Part model, mm, in its own coordinate system. A direction names the side the tool comes from. Give positions to 0.01 mm unless a question says otherwise; leave off trailing zeros. Order: outer loops, then holes, each group sorted by start corner. A loop starts at its lowest first (then second) coordinate and runs counter-clockwise, first axis right, second up.
from build123d import *

# Parameters (mm, degrees)
BOSS_EXTRUDE1_DEPTH   = 5.588
F_6_CLEARANCE_HOLE1_D = 3.7973
M2_CLEARANCE_HOLE1_D  = 2.4
CUT_EXTRUDE1_REACH    = 254.133
SKETCH8_R             = 5.08


with BuildPart() as part:
    # Sketch1 → Boss-Extrude1 (new body)
    with BuildSketch(Plane(origin=(0, 0, 0), x_dir=(1, 0, 0), z_dir=(0, 1, 0))):
        with BuildLine():
            Line((12.7, 72.898), (31.75, 72.898))
            Line((31.75, 72.898), (31.75, 67.056))
            Line((31.75, 67.056), (44.45, 67.056))
            Line((44.45, 67.056), (44.45, 72.898))
            Line((44.45, 72.898), (69.85, 72.898))
            Line((69.85, 72.898), (69.85, 67.31))
            Line((69.85, 67.31), (114.3, 67.31))
            Line((114.3, 67.31), (114.3, 72.898))
            Line((114.3, 72.898), (139.7, 72.898))
            Line((139.7, 72.898), (139.7, 67.31))
            Line((139.7, 67.31), (165.1, 67.31))
            Line((165.1, 67.31), (165.1, 72.898))
            Line((165.1, 72.898), (190.5, 72.898))
            Line((190.5, 72.898), (190.5, 67.056))
            Line((190.5, 67.056), (222.25, 67.056))
            Line((222.25, 67.056), (222.25, 72.898))
            Line((222.25, 72.898), (241.3, 72.898))
            Line((241.3, 72.898), (241.3, 0))
            Line((241.3, 0), (171.45, 0))
            ThreePointArc((171.45, 0), (162.469743879, -3.719743879), (158.75, -12.7))
            Line((158.75, -12.7), (158.75, -42.164))
            Line((158.75, -42.164), (146.05, -42.164))
            Line((146.05, -42.164), (146.05, 0.122766638))
            Line((146.05, 0.122766638), (127, 0.122766638))
            Line((127, 0.122766638), (107.95, 0.122766638))
            Line((107.95, 0.122766638), (107.95, -42.164))
            Line((107.95, -42.164), (95.25, -42.164))
            Line((95.25, -42.164), (95.25, -12.7))
            ThreePointArc((95.25, -12.7), (91.530256121, -3.719743879), (82.55, 0))
            Line((82.55, 0), (12.7, 0))
            Line((12.7, 0), (12.7, 72.898))
        make_face()
    extrude(amount=BOSS_EXTRUDE1_DEPTH)

    # #6 Clearance Hole1 (through all)
    with Locations(Plane(origin=(0, 0, 0), x_dir=(-1, 0, 0), z_dir=(0, -1, 0))):
        with Locations((-102.362, -32.397617544), (-151.638, -32.397617544), (-151.638, -5.456849181), (-102.362, -5.456849181)):
            Hole(F_6_CLEARANCE_HOLE1_D / 2)

    # M2 Clearance Hole1 (through all)
    with Locations(Plane(origin=(0, 5.588, 0), x_dir=(1, 0, 0), z_dir=(0, 1, 0))):
        with Locations((33.528, 58.166), (53.848, 58.166), (53.848, 37.846), (33.528, 37.846)):
            Hole(M2_CLEARANCE_HOLE1_D / 2)

    # Sketch8 → Cut-Extrude1 (cut, up to next)
    with BuildSketch(Plane(origin=(0, 5.588, 0), x_dir=(1, 0, 0), z_dir=(0, 1, 0)), mode=Mode.PRIVATE) as cut_extrude1_sk1:
        with Locations(Location((28.448, 15.870766638, 0), (0, 0, 270))):
            Circle(SKETCH8_R)
    cut_extrude1_tool1 = extrude(cut_extrude1_sk1.sketch, amount=-CUT_EXTRUDE1_REACH, mode=Mode.PRIVATE) & part.part
    # Sketch8 → Cut-Extrude1 (cut, up to next)
    with BuildSketch(Plane(origin=(0, 5.588, 0), x_dir=(1, 0, 0), z_dir=(0, 1, 0)), mode=Mode.PRIVATE) as cut_extrude1_sk2:
        with Locations(Location((225.552, 15.870766638, 0), (0, 0, 270))):
            Circle(SKETCH8_R)
    cut_extrude1_tool2 = extrude(cut_extrude1_sk2.sketch, amount=-CUT_EXTRUDE1_REACH, mode=Mode.PRIVATE) & part.part
    add(cut_extrude1_tool1.solids().sort_by_distance((28.448, 5.588, -15.870767))[0], mode=Mode.SUBTRACT)
    add(cut_extrude1_tool2.solids().sort_by_distance((225.552, 5.588, -15.870767))[0], mode=Mode.SUBTRACT)


solid = part.part
Item 1: Pull direction Z, two halves, no side cores. Call faces 1 (the face through (31.9, 2.8, -19.6)), 2 (the face through (241.3, 3, -37)), 3 (the face through (48, 3, 0)): released by +Z, released by -Z, zero draft, split by the parting line, or undercut.
Item 2: Drill centre lines: probe 1 along X at (y, z) = (2.9, -57.5); probe 2 along X at (y, z) = (1.95, 35.5); probe 3 along X at (y, z) = (5, -17.5). Where is each one in solid material? Low to high.
Item 3: Band-saw the part on B-B on x = 144. List the corners of the cut face in (y, z), plus the area to 3 significant figures.
Item 4: Band-saw the part on C-C on y = 3. Give the number of separate pieces and of enclosed holes in the cut face, plus the area to 3 significant figures.
Item 5: Which spindle directions (+Z, -Z, +X, -X, +Y, -Y) get a long thin tool onto all of the face, cutting with end or side? Do faces 4 (the face through (207, 3, 0)), 5 (the face through (31.75, 3, -70)), 6 (the face through (146.05, 3, 21)). Say none if no direction does.
Item 6: Band-saw the part on D-D on x = 118. List the corners of the cut face in (y, z), plus the area to 3 significant figures.
Item 7: Drop flat-ended pins along their axis: P1, Ø3, axis at x = 203, y = 4, coming from the +Z side; P2, Ø1.7, axis at x = 36.5, y = 1.5, coming from the -Z side; P3, Ø3, axis at y = 2, z = 31.5, coming from the -X side. Give the stop position or say it passes through.
Item 8: Band-saw the part on A-A on z = 18.5. List the corners of the cut face in (x, y), plus the area to 3 significant figures.
Working result:
1. face 1: undercut
1. face 2: zero draft
1. face 3: released by +Z
2. probe 1: x = 12.7 to 32.53, 34.53 to 52.85, 54.85 to 241.3
2. probe 2: x = 95.25 to 107.95, 146.05 to 158.75
2. probe 3: x = 12.7 to 23.64, 33.26 to 220.74, 230.36 to 241.3
3. outline: (0, -67.31) - (5.59, -67.31) - (5.59, -0.12) - (0, -0.12) - close
3. area: 375 mm2
4. separate pieces: 1
4. enclosed holes: 10
4. area: 16,900 mm2
5. face 4: +Z, +X, +Y, -Y
5. face 5: -Z, +Y, -Y
5. face 6: +Z, +Y, -Y
6. outline: (0, -72.9) - (5.59, -72.9) - (5.59, -0.12) - (0, -0.12) - close
6. area: 407 mm2
7. P1: stops at z = 0
7. P2: stops at z = -67.06
7. P3: stops at x = 95.25
8. outline: (95.25, 0) - (107.95, 0) - (107.95, 5.59) - (95.25, 5.59) - close; (146.05, 0) - (158.75, 0) - (158.75, 5.59) - (146.05, 5.59) - close
8. area: 142 mm2
